Here's the drawing with two shaded views (mm, measured from the low corner). I have some questions. A direction names the side the tool comes from. Give positions to 0.01 mm unless a question says otherwise; leave off trailing zeros. Loops run counter-clockwise (first coordinate to the right, second up) from the corner with the lowest first, then second, coordinate; pieces in that order, holes last. Notation, with made-up numbers: (63, -18) - (116, -18) arc R30 ccw to (116, 11) - close; hole circle Ø1 at (3.25, 37.25). An arc over 180 degrees is marked (long way). Use a Markdown table: item, result. Add a question column.
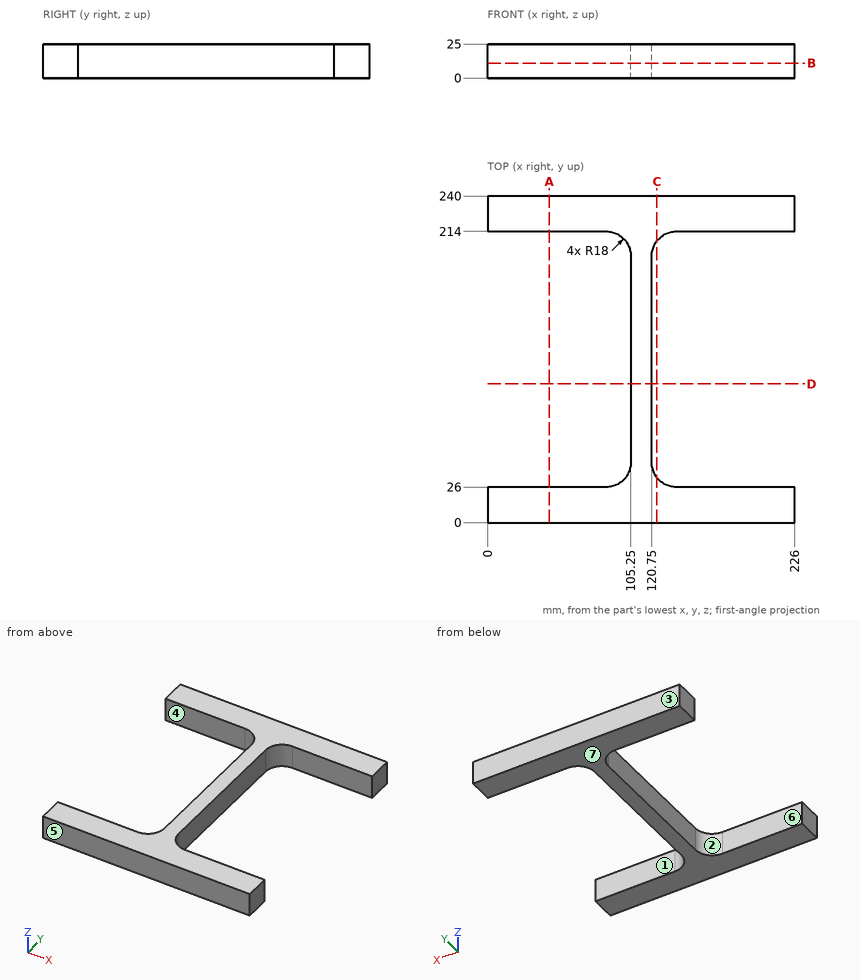
1. Please list where these lines run through material, in increasing order: line 1 along Y through (x, z) = (173, 12.75); line 2 along X through (y, z) = (132, 8); line 3 along Y through (x, z) = (123, 3). Write a range as [from, to].
2. Suppose I cut it at C-C (x = 124.5). List the corners of the cut face in (y, z) for me, and give its area (3 significant figures).
3. On a 3-axis mill with a long thin cutter (end or side, diameter ignored), from which of +Z, -Z, +X, -X, +Y, -Y can I reach the whole of each face in a straight line? I mean the marked faces 1, 2 and 3. Say none if no direction works.
4. Suppose I cut it at A-A (x = 45.5). List the corners of the cut face in (y, z) for me.
5. Will these pins go through, and if not, where does the flat tip stop? P1, Ø10, axis at y = 40.5, z = 6.5, coming from the +X side; P2, Ø4, axis at y = 57, z = 16.5, coming from the -X side; P3, Ø6, axis at y = 192.5, z = 18.5, coming from the +X side.
6. Suppose I cut it at D-D (y = 102). List the corners of the cut face in (x, z) for me, and give its area (4 significant figures).
7. Suppose I cut it at B-B (z = 11). List the corners of the cut face in (x, y) for me, and give its area (3 significant figures).
8. If we mould it in two halves opening along Y, with no side actions, what happens to the marked faces 4, 5, 6 and 7? For each: released by +Y, released by -Y, zero draft, split by the parting line, or undercut.
Results below:
| question | item | result |
|---|---|---|
| 1 | line 1 | [0, 26], [214, 240] |
| 1 | line 2 | [105.25, 120.75] |
| 1 | line 3 | [0, 35.29], [204.71, 240] |
| 2 | outline | (0, 0) - (33, 0) - (33, 25) - (0, 25) - close; (207, 0) - (240, 0) - (240, 25) - (207, 25) - close |
| 2 | area | 1,650 mm² |
| 3 | face 1 | +Z, -Z, +X |
| 3 | face 2 | +Z, -Z, -X |
| 3 | face 3 | +Z, -Z, +X, -X, +Y |
| 4 | outline | (0, 0) - (26, 0) - (26, 25) - (0, 25) - close; (214, 0) - (240, 0) - (240, 25) - (214, 25) - close |
| 5 | P1 | x = 122.88 |
| 5 | P2 | x = 105.25 |
| 5 | P3 | x = 120.75 |
| 6 | outline | (105.25, 0) - (120.75, 0) - (120.75, 25) - (105.25, 25) - close |
| 6 | area | 387.5 mm² |
| 7 | outline | (0, 0) - (226, 0) - (226, 26) - (138.75, 26) arc R18 cw to (120.75, 44) - (120.75, 196) arc R18 cw to (138.75, 214) - (226, 214) - (226, 240) - (0, 240) - (0, 214) - (87.25, 214) arc R18 cw to (105.25, 196) - (105.25, 44) arc R18 cw to (87.25, 26) - (0, 26) - close |
| 7 | area | 14,900 mm² |
| 8 | face 4 | undercut |
| 8 | face 5 | released by -Y |
| 8 | face 6 | undercut |
| 8 | face 7 | zero draft |
